Build history of the part. All positions in model axes, mm. Coordinates: 2 decimals unless noted, no trailing zeros. Write each loop counter-clockwise with the first axis right and the second up, starting at its lowest first coordinate (ties: lowest second). Pieces come first, ordered by that corner, then holes.
```python
from build123d import *

# Parameters (mm, degrees)
SKETCH1_W   = 34
SKETCH1_H   = 35
SKETCH1_R   = 1.5
BOARD_DEPTH = 1.5
SKETCH2_R   = 0.9
SKETCH2_R_2 = 0.5
HOLES_DEPTH = 2


with BuildPart() as part:
    # Sketch1 → Board (new body)
    with BuildSketch(Plane.XY):
        Rectangle(SKETCH1_W, SKETCH1_H)
        with Locations((-14.5, 15)):
            Circle(SKETCH1_R, mode=Mode.SUBTRACT)
        with Locations((-14.5, -15)):
            Circle(SKETCH1_R, mode=Mode.SUBTRACT)
        with Locations((14.5, -15)):
            Circle(SKETCH1_R, mode=Mode.SUBTRACT)
        with Locations((14.5, 15)):
            Circle(SKETCH1_R, mode=Mode.SUBTRACT)
    extrude(amount=BOARD_DEPTH)

    # Sketch2 → Holes (cut)
    with BuildSketch(Plane(origin=(0, 0, 0), x_dir=(-1, 0, 0), z_dir=(0, 0, -1))):
        with Locations((-10, 4.5)):
            Circle(SKETCH2_R)
        with Locations((10, 4.5)):
            Circle(SKETCH2_R)
        with Locations((10.16, -9.69)):
            Circle(SKETCH2_R_2)
        with Locations((10.16, -12.23)):
            Circle(SKETCH2_R_2)
        with Locations((7.62, -12.23)):
            Circle(SKETCH2_R_2)
        with Locations((7.62, -9.69)):
            Circle(SKETCH2_R_2)
        with Locations((5.08, -12.23)):
            Circle(SKETCH2_R_2)
        with Locations((5.08, -9.69)):
            Circle(SKETCH2_R_2)
        with Locations((2.54, -12.23)):
            Circle(SKETCH2_R_2)
        with Locations((2.54, -9.69)):
            Circle(SKETCH2_R_2)
        with Locations((0, -12.23)):
            Circle(SKETCH2_R_2)
        with Locations((0, -9.69)):
            Circle(SKETCH2_R_2)
        with Locations((-2.54, -12.23)):
            Circle(SKETCH2_R_2)
        with Locations((-2.54, -9.69)):
            Circle(SKETCH2_R_2)
        with Locations((-5.08, -12.23)):
            Circle(SKETCH2_R_2)
        with Locations((-5.08, -9.69)):
            Circle(SKETCH2_R_2)
        with Locations((-7.62, -12.23)):
            Circle(SKETCH2_R_2)
        with Locations((-7.62, -9.69)):
            Circle(SKETCH2_R_2)
        with Locations((-10.16, -12.23)):
            Circle(SKETCH2_R_2)
        with Locations((-10.16, -9.69)):
            Circle(SKETCH2_R_2)
    extrude(amount=-HOLES_DEPTH, mode=Mode.SUBTRACT)


solid = part.part
```
1. Mould opens along X. For faces 1 (the face through (0, 0, 1.5)), 2 (the face through (-17, 0, 1)), 3 (the face through (-2.81, -9.27, 0.74)) say: +X half, -X half, draft (parallel to the pull), parting line (faces both ways), or undercut.
Computed values:
face 1: draft
face 2: -X half
face 3: undercut
2. Saw through at B-B on x = 14.5. List the corners of the cut face in (y, z).
Computed values:
outline: (-17.5, 0) - (-16.5, 0) - (-16.5, 1.5) - (-17.5, 1.5) - close; (-13.5, 0) - (13.5, 0) - (13.5, 1.5) - (-13.5, 1.5) - close; (16.5, 0) - (17.5, 0) - (17.5, 1.5) - (16.5, 1.5) - close
3. Saw through at C-C on z = 0.25. State how many separate pieces and enclosed holes the cut face has, plus the area to 3 significant figures.
Computed values:
separate pieces: 1
enclosed holes: 24
area: 1,140 mm2
4. Probe line 1 along Y through (x, z) = (0, 0.55); line 2 along Y through (x, z) = (14.5, 0.5); line 3 along X through (y, z) = (16, 0.4). List the from-to ranges inside material, lowest first.
Computed values:
line 1: y = -17.5 to -12.73, -11.73 to -10.19, -9.19 to 17.5
line 2: y = -17.5 to -16.5, -13.5 to 13.5, 16.5 to 17.5
line 3: x = -17 to -15.62, -13.38 to 13.38, 15.62 to 17
5. Saw through at D-D on x = 10.16. List the corners of the cut face in (y, z).
Computed values:
outline: (-17.5, 0) - (-12.73, 0) - (-12.73, 1.5) - (-17.5, 1.5) - close; (-11.73, 0) - (-10.19, 0) - (-10.19, 1.5) - (-11.73, 1.5) - close; (-9.19, 0) - (3.61, 0) - (3.61, 1.5) - (-9.19, 1.5) - close; (5.39, 0) - (17.5, 0) - (17.5, 1.5) - (5.39, 1.5) - close
6. Saw through at A-A on y = -15. List the corners of the cut face in (x, z), plus the area to 3 significant figures.
Computed values:
outline: (-17, 0) - (-16, 0) - (-16, 1.5) - (-17, 1.5) - close; (-13, 0) - (13, 0) - (13, 1.5) - (-13, 1.5) - close; (16, 0) - (17, 0) - (17, 1.5) - (16, 1.5) - close
area: 42.0 mm2
